from build123d import *

# Parameters (mm, degrees)
SKETCH_1_R          = 38
SKETCH_1_R_2        = 30
EXTRUDE_1_DEPTH     = 10
SKETCH_2_W          = 8
SKETCH_2_H          = 60
EXTRUDE_2_DEPTH     = 80
SKETCH_3_R          = 4
CUT_EXTRUDE_1_DEPTH = 80
SKETCH_4_W          = 60
SKETCH_4_H          = 40.678120155
CUT_EXTRUDE_2_DEPTH = 81
EXTRUDE_3_DEPTH     = 24
SKETCH_7_W          = 8
SKETCH_7_H          = 16
EXTRUDE_5_DEPTH     = 16
CUT_EXTRUDE_3_DEPTH = 81


with BuildPart() as part:
    # 草图1 → 凸台-拉伸1 (new body)
    with BuildSketch(Plane(origin=(0, 0, 0), x_dir=(1, 0, 0), z_dir=(0, 1, 0))):
        Circle(SKETCH_1_R)
        Circle(SKETCH_1_R_2, mode=Mode.SUBTRACT)
    extrude(amount=EXTRUDE_1_DEPTH)

    # 草图2 → 凸台-拉伸2 (add)
    with BuildSketch(Plane.XZ):
        with Locations((-34, 0)):
            Rectangle(SKETCH_2_W, SKETCH_2_H)
        with Locations((34, 0)):
            Rectangle(SKETCH_2_W, SKETCH_2_H)
    extrude(amount=-EXTRUDE_2_DEPTH)

    # 草图3 → 切除-拉伸1 (cut)
    with BuildSketch(Plane(origin=(38, 0, 0), x_dir=(0, 0, -1), z_dir=(1, 0, 0))):
        with Locations((0, 50)):
            Circle(SKETCH_3_R)
        with BuildLine():
            Line((-30, 50), (-30, 88))
            Line((-30, 88), (30, 88))
            Line((30, 88), (30, 50))
            ThreePointArc((30, 50), (0, 80), (-30, 50))
        make_face()
    extrude(amount=-CUT_EXTRUDE_1_DEPTH, mode=Mode.SUBTRACT)

    # 草图4 → 切除-拉伸2 (cut, through all)
    with BuildSketch(Plane.XZ):
        with Locations((0, -20.339060078)):
            Rectangle(SKETCH_4_W, SKETCH_4_H)
    extrude(amount=-CUT_EXTRUDE_2_DEPTH, mode=Mode.SUBTRACT)

    # 草图5 → 凸台-拉伸3 (add)
    with BuildSketch(Plane(origin=(0, 10, 0), x_dir=(1, 0, 0), z_dir=(0, 1, 0))):
        with BuildLine():
            Line((42, 0), (38, 0))
            ThreePointArc((38, 0), (0, -38), (-38, 0))
            Line((-38, 0), (-42, 0))
            ThreePointArc((-42, 0), (0, -42), (42, 0))
        make_face()
    extrude(amount=-EXTRUDE_3_DEPTH)

    # 草图7 → 凸台-拉伸5 (add)
    with BuildSketch(Plane.XY.offset(30)):
        with Locations((-34, 28)):
            Rectangle(SKETCH_7_W, SKETCH_7_H)
        with Locations((34, 28)):
            Rectangle(SKETCH_7_W, SKETCH_7_H)
    extrude(amount=EXTRUDE_5_DEPTH)

    # 草图8 → 切除-拉伸3 (cut, through all)
    with BuildSketch(Plane(origin=(38, 0, 0), x_dir=(0, 0, -1), z_dir=(1, 0, 0))):
        with BuildLine():
            Line((-38, 36), (-49.79015057, 36))
            Line((-49.79015057, 36), (-49.79015057, 20))
            Line((-49.79015057, 20), (-38, 20))
            ThreePointArc((-38, 20), (-46, 28), (-38, 36))
        make_face()
    extrude(amount=-CUT_EXTRUDE_3_DEPTH, mode=Mode.SUBTRACT)


solid = part.part
Read the model definition and answer for the solid it produces. Units are mm, in the model's axes. A direction names the side the tool comes from. Give positions to 0.01 mm unless a question says otherwise; leave off trailing zeros. Write each loop counter-clockwise with the first axis right and the second up, starting at its lowest first coordinate (ties: lowest second). Pieces come first, ordered by that corner, then holes. Notation, with made-up numbers: (-16, 62.25) - (10, 62.25) arc R24 ccw to (10, 82.25) - close; hole circle Ø8 at (33, -38). An arc over 180 degrees is marked (long way). Answer in a Markdown table with one row per item. Add a question column.
Item 1: Section C-C, the plane x = -33.5 is taken. Write down the section's boundary in (y, z).
Item 2: Flat-ended cylindrical pins translate along their axes: P1, Ø9, axis at x = 33.5, y = 43, coming from the +Z side; P2, Ø4, axis at x = 35.5, z = 25, coming from the -Y side; P3, Ø12, axis at y = 37.5, z = 13.5, coming from the +X side; P4, Ø4, axis at x = 33, z = 34.5, coming from the -Y side. Find the tip coordinate at first contact, or state that the pin passes through.
Item 3: Section A-A, the plane y = 28 is taken. Write down the section's boundary in (x, z).
Item 4: Section D-D, the plane z = 32.5 is taken. Write down the section's boundary in (x, y).
Item 5: Section B-B, the plane z = 22 is taken. Write down the section's boundary in (x, y), and give its area (3 significant figures).
Item 6: Determine the mould class of faces 5 (the face through (34, 10, 30)), 6 (the face through (-30, 39, -1)), 7 (the face through (34.056, 46.095, 0.867)) for opening direction Z: pulls with the +Z half, pulls with the -Z half, needs draft (parallel to the pull), parting line crosses it, or undercut.
Item 7: Find the intervals of material crossed by L1, parallel to Y at x = 31, z = 0; L2, parallel to X at y = 23, z = 26; L3, parallel to X at y = 5.5, z = 0.5, in increasing order.
Item 8: A tool of negligible diameter and unlimited length cuts with its end or side. For faces 1 (the face through (-40, 10, 7)), 2 (the face through (-34, 10, 30)), 3 (the face through (35, 0, 27)), 4 (the face through (34, 36, 34)), from which of +Z, -Z, +X, -X, +Y, -Y can it reach the whole face along a straight path? Write none if from no direction.
Recorded:
| question | item | result |
|---|---|---|
| 1 | outline | (-14, 17.94) - (0, 17.94) - (0, -30) - (50, -30) arc R30 ccw to (50, 30) - (36, 30) - (36, 38) arc R8 ccw to (20, 38) - (20, 30) - (0, 30) - (0, 25.33) - (-14, 25.33) - close; hole circle Ø8 at (50, 0) |
| 2 | P1 | stops at z = 30 |
| 2 | P2 | stops at y = -14 |
| 2 | P3 | stops at x = 38 |
| 2 | P4 | stops at y = 20 |
| 3 | outline | (-38, -30) - (-30, -30) - (-30, 46) - (-38, 46) - close; (30, -30) - (38, -30) - (38, 46) - (30, 46) - close |
| 4 | outline | (-38, 20) - (-30, 20) - (-30, 36) - (-38, 36) - close; (-26.6, -14) - (-19.69, -14) - (-19.69, 0) - (19.69, 0) - (19.69, -14) - (26.6, -14) - (26.6, 10) - (-26.6, 10) - close; (30, 20) - (38, 20) - (38, 36) - (30, 36) - close |
| 5 | outline | (-38, 0) - (-35.78, 0) - (-35.78, -14) - (-30.98, -14) - (-30.98, 0) - (-20.4, 0) - (-20.4, 10) - (-30, 10) - (-30, 70.4) - (-38, 70.4) - close; (20.4, 0) - (30.98, 0) - (30.98, -14) - (35.78, -14) - (35.78, 0) - (38, 0) - (38, 70.4) - (30, 70.4) - (30, 10) - (20.4, 10) - close |
| 5 | area | 1,450 mm2 |
| 6 | face 5 | pulls with the +Z half |
| 6 | face 6 | needs draft |
| 6 | face 7 | undercut |
| 7 | L1 | y = 0 to 46, 54 to 80 |
| 7 | L2 | x = -38 to -30, 30 to 38 |
| 7 | L3 | x = -42 to -30, 30 to 42 |
| 8 | face 1 | +Z, -Z, -X, +Y |
| 8 | face 2 | +Z, -X, -Y |
| 8 | face 3 | +Z, +X, -Y |
| 8 | face 4 | +Z, +X, -X, +Y |
